Source: CAD feature listing. Evaluate the final solid. Frame: model axes, mm. A direction names the side the tool comes from. Give positions to 0.01 mm unless a question says otherwise; leave off trailing zeros. Loops run counter-clockwise (first coordinate to the right, second up) from the corner with the lowest first, then second, coordinate; pieces in that order, holes last. Notation, with made-up numbers: M 86,-35 L 136,-35 A28 cw 136,2 Z; hole C 20,52.5 d3. An arc over 180 degrees is marked long. Answer in a Markdown table with one row per item.
```python
from build123d import *

# Parameters (mm, degrees)
F0_W     = 113.3312
F0_H     = 139.3312
F1_DEPTH = 13
F3_DEPTH = 8


# Not quite as in the source:
# - ends of sketch curves that miss each other by under 0.0002 mm in the source are joined


with BuildPart() as f1:
    # F0 (on Top) → F1 (new body)
    with BuildSketch(Plane.XY):
        Rectangle(F0_W, F0_H)
    extrude(amount=F1_DEPTH)

    # F2 (on face) → F3 (cut)
    with BuildSketch(Plane.XY.offset(13)):
        with BuildLine():
            Line((26.3344, -49.6656), (36.6656, -49.6656))
            Line((36.6656, -49.6656), (36.665598632, -26.6656016949))
            Line((36.665598632, -26.6656016949), (46.6656, -26.6656))
            Line((46.6656, -26.6656), (46.665598632, -6.6656015976))
            Line((46.665598632, -6.6656015976), (36.6656, -6.6656))
            Line((36.6656, -6.6656), (36.6655984, 35.3343984024))
            ThreePointArc((36.6655984, 35.3343984024), (27.823544274, 48.5726978027), (12.2081110977, 45.4754831032))
            Line((12.2081110977, 45.4754831032), (-30.4382024275, 4.5465657527))
            ThreePointArc((-30.4382024275, 4.5465657527), (-35.0404373732, -1.9072796936), (-36.6656, -9.6656))
            Line((-36.6656, -9.6656), (-36.6656, -16.6656))
            Line((-36.6656, -16.6656), (-36.6656, -49.6656))
            Line((-36.6656, -49.6656), (-26.3344000004, -49.6656))
            Line((-26.3344000004, -49.6656), (-26.3344000004, -16.6656))
            Line((-26.3344000004, -16.6656), (-26.3344000004, -9.6656))
            ThreePointArc((-26.3344000004, -9.6656), (-25.6512318575, -6.2260785418), (-23.7054426981, -3.3087285252))
            ThreePointArc((-23.7054426981, -3.3087285252), (-23.7019028512, -3.3051827615), (-23.6983610309, -3.3016389689))
            ThreePointArc((-23.6983610309, -3.3016389689), (-23.566271734, -3.172236103), (-23.4315517652, -3.0455742931))
            Line((-23.4315517652, -3.0455742931), (-11.3959568303, 8.5053390806))
            Line((-11.3959568303, 8.5053390806), (-11.220990014, 8.6732598648))
            Line((-11.220990014, 8.6732598648), (-11.2208270158, 8.6734162989))
            Line((-11.2208270158, 8.6734162989), (9.6364044846, 28.6907129577))
            Line((9.6364044846, 28.6907129577), (9.6666794098, 28.7197686911))
            Line((9.6666794098, 28.7197686911), (19.3337239366, 37.9975147862))
            Line((19.3337239366, 37.9975147862), (19.5059733761, 38.162827624))
            ThreePointArc((19.5059733761, 38.162827624), (23.8651336494, 39.0299159917), (26.334398632, 35.3343983051))
            Line((26.334398632, 35.3343983051), (26.334398632, -6.6656016949))
            Line((26.334398632, -6.6656016949), (16.3344, -6.6656))
            Line((16.3344, -6.6656), (16.334398632, -26.6656016949))
            Line((16.334398632, -26.6656016949), (26.3344, -26.6656))
            Line((26.3344, -26.6656), (26.3344, -49.6656))
        make_face()
        with BuildLine():
            ThreePointArc((-30.988946, 4.018001), (-30.7197680452, 4.2814242377), (-30.4455091202, 4.5395533054))
            Line((-30.4455091202, 4.5395533054), (-30.988946, 4.018001))
        make_face(mode=Mode.SUBTRACT)
        with BuildLine():
            Line((-30.988946, 4.018001), (-30.4455091202, 4.5395533054))
            ThreePointArc((-30.4455091202, 4.5395533054), (-30.7197680452, 4.2814242377), (-30.988946, 4.018001))
        make_face()
        with BuildLine():
            Line((-23.6983610309, -3.3016389689), (-23.4315517652, -3.0455742931))
            ThreePointArc((-23.4315517652, -3.0455742931), (-23.566271734, -3.172236103), (-23.6983610309, -3.3016389689))
        make_face()
        with BuildLine():
            ThreePointArc((-11.2206003272, 8.6733407274), (-11.2207136714, 8.6733785135), (-11.2208270158, 8.6734162989))
            Line((-11.2208270158, 8.6734162989), (-11.220990014, 8.6732598648))
            ThreePointArc((-11.220990014, 8.6732598648), (-11.220876669, 8.6732220799), (-11.2207633243, 8.6731842943))
            Line((-11.2207633243, 8.6731842943), (-11.2206003272, 8.6733407274))
        make_face()
    extrude(amount=-F3_DEPTH, mode=Mode.SUBTRACT)


solid = f1.part
```
Q1. Reachability of faces 4 (the flat face through (42, -6.666, 9)), 5 (the flat face through (-1, 1, 0)) from +Z, -Z, +X, -X, +Y, -Y: full face, straight path, thin tool, end or side. Return the list, or none.
Values follow:
| item | result |
|---|---|
| face 4 | +Z |
| face 5 | -Z, +X, -X, +Y, -Y |
Q2. Section query C-C (x = -13). Output: boundary loops of the cut face in (y, z), plus the area to 3 significant figures.
Values follow:
| item | result |
|---|---|
| outline | M -69.67,0 L 69.67,0 L 69.67,13 L 21.28,13 L 21.28,5 L 6.97,5 L 6.97,13 L -69.67,13 Z |
| area | 1,700 mm^2 |
Q3. Section query B-B (y = -34). Output: boundary loops of the cut face in (x, z), plus the area to 3 significant figures.
Values follow:
| item | result |
|---|---|
| outline | M -56.67,0 L 56.67,0 L 56.67,13 L 36.67,13 L 36.67,5 L 26.33,5 L 26.33,13 L -26.33,13 L -26.33,5 L -36.67,5 L -36.67,13 L -56.67,13 Z |
| area | 1,310 mm^2 |
Q4. Mould query, pull axis X, two halves, no side actions, for faces 1 (the flat face through (26.334, -38, 9)), 2 (the flat face through (-1, -69.666, 6)), 3 (the flat face through (-56.666, -1, 6)). Classes: +X half, -X half, draft (parallel to the pull), parting line (faces both ways), or undercut.
Values follow:
| item | result |
|---|---|
| face 1 | undercut |
| face 2 | draft |
| face 3 | -X half |
Q5. Ray query, probe 1 along X at (y, z) = (-47.5, 5.75); probe 2 along X at (y, z) = (-16, 10.5); probe 3 along Y at (x, z) = (25.5, 12.75). Return the intervals inside material, ascending. Write a range as from..to.
Values follow:
| item | result |
|---|---|
| probe 1 | -56.67..-36.67, -26.33..26.33, 36.67..56.67 |
| probe 2 | -56.67..-36.67, -26.33..16.33, 46.67..56.67 |
| probe 3 | -69.67..-26.67, -6.67..37.78, 49.31..69.67 |
Q6. Section query D-D (y = 22). Output: boundary loops of the cut face in (x, z), plus the area to 3 significant figures.
Values follow:
| item | result |
|---|---|
| outline | M -56.67,0 L 56.67,0 L 56.67,13 L 36.67,13 L 36.67,5 L 26.33,5 L 26.33,13 L 2.66,13 L 2.66,5 L -12.25,5 L -12.25,13 L -56.67,13 Z |
| area | 1,270 mm^2 |
